from build123d import *

# Parameters (mm, degrees)
F0_R          = 11.049
F1_DEPTH      = 76.2
F1_DEPTH_BACK = 76.2
F2_W          = 61.722
F2_H          = 152.4
F3_DEPTH      = 101.6
F4_T          = -2.54


with BuildPart() as f1:
    # F0 (on Front) → F1 (new body, two sides)
    with BuildSketch(Plane.XZ) as f1_sk:
        with BuildLine():
            ThreePointArc((10.170598, -40.91247), (11.863519, -37.501733), (12.446, -33.738778))
            ThreePointArc((12.446, -33.738778), (-3.762954, -21.875259), (-10.170598, -40.91247))
            ThreePointArc((-10.170598, -40.91247), (0, -46.184778), (10.170598, -40.91247))
        make_face()
        with Locations((0, -33.738778)):
            Circle(F0_R, mode=Mode.SUBTRACT)
        with BuildLine():
            ThreePointArc((-10.170598, -40.91247), (-3.762954, -21.875259), (12.446, -33.738778))
            ThreePointArc((12.446, -33.738778), (11.863519, -37.501733), (10.170598, -40.91247))
            Line((10.170598, -40.91247), (30.861, -11.578374))
            Line((30.861, -11.578374), (0, -11.578374))
            Line((0, -11.578374), (-30.861, -11.578374))
            Line((-30.861, -11.578374), (-10.170598, -40.91247))
        make_face()
    extrude(amount=F1_DEPTH)
    extrude(f1_sk.sketch, amount=-F1_DEPTH_BACK)

    # F2 (on face) → F3 (join)
    with BuildSketch(Plane.XY.offset(-11.578374)):
        Rectangle(F2_W, F2_H)
    extrude(amount=F3_DEPTH)

    # F4
    f4_openings = [f1.faces().sort_by_distance(p)[0] for p in [
        (0, 0, 90.021626),
    ]]
    offset(amount=F4_T, openings=f4_openings)


solid = f1.part
Design review of the part built by this model. Coordinates are the model's own, in mm. A direction names the side the tool comes from. Coordinates: 2 decimals unless noted, no trailing zeros. Write each loop counter-clockwise with the first axis right and the second up, starting at its lowest first coordinate (ties: lowest second). Pieces come first, ordered by that corner, then holes. Notation, with made-up numbers: (7, -36) -> (65, -36) arc R12 ccw to (65, -24) -> close; hole circle Ø1 at (33.5, -13.75). An arc over 180 degrees is marked (long way). Write each question's results on one line, items separated by ' | '. Start each with the question number.
(1) The part is to be moulded in two halves that separate along Z. For faces 3 (the face through (-30, 23, 90.022)), 4 (the face through (0, -76.2, 36)), 5 (the face through (-1.438, 1.067, -22.784)), say which applies: pulls with the +Z half, pulls with the -Z half, needs draft (parallel to the pull), parting line crosses it, or undercut.
(2) Clearance check with flat-ended pins moving along their axes: P1, Ø12, axis at x = 18.5, y = -20.5, coming from the +Z side; P2, Ø4, axis at x = -18, y = 3.5, coming from the +Z side; P3, Ø6, axis at x = 9.5, y = 7.5, coming from the -Z side. State where each tip first meets the part, or that it passes through.
(3) Take a section at D-D on z = -5. Write out the cut boundary in (x, y).
(4) Tool access review of faces 1 (the face through (-0.167, -1.067, -46.184)), 2 (the face through (20.785, -1.031, -21.457)): name each direction out of +Z, -Z, +X, -X, +Y, -Y from which nothing blocks a thin tool from reaching the whole face with its end or side.
(5) Take a section at A-A on x = 0. Write out the cut boundary in (y, z), and give its area (3 significant figures).
(6) Take a section at C-C on y = 50. Write out the cut boundary in (x, z).
(7) For line 1 along Y through (x, z) = (-13, 8); line 2 along X through (y, z) = (-28.5, 34.5); line 3 along Z through (x, y) = (0, 1.5), list the stretches that pass through material, from the lowest coordinate up. Write a range as from..to.
(8) Take a section at B-B on z = -25.5. Write out the cut boundary in (x, y), and give its area (3 significant figures).
Results found:
1) face 3: pulls with the +Z half | face 4: needs draft | face 5: undercut
2) P1: stops at z = -16.19 | P2: stops at z = -22.57 | P3: stops at z = -44.35
3) outline: (-30.86, -76.2) -> (30.86, -76.2) -> (30.86, 76.2) -> (-30.86, 76.2) -> close; hole (-28.32, -73.66) -> (28.32, -73.66) -> (28.32, 73.66) -> (-28.32, 73.66) -> close
4) face 1: -Z, +Y, -Y | face 2: +Z
5) outline: (-76.2, -46.18) -> (76.2, -46.18) -> (76.2, -44.79) -> (-76.2, -44.79) -> close; (-76.2, -22.69) -> (76.2, -22.69) -> (76.2, 90.02) -> (73.66, 90.02) -> (73.66, -20.15) -> (-73.66, -20.15) -> (-73.66, 90.02) -> (-76.2, 90.02) -> close | area: 1,160 mm2
6) outline: (-30.86, -11.58) -> (-10.17, -40.91) arc R12.45 ccw to (10.17, -40.91) -> (30.86, -11.58) -> (30.86, 90.02) -> (28.32, 90.02) -> (28.32, -10.77) -> (13.46, -31.85) arc R13.59 ccw to (-13.46, -31.85) -> (-28.32, -10.77) -> (-28.32, 90.02) -> (-30.86, 90.02) -> close; hole circle Ø22.1 at (0, -33.74)
7) line 1: y = -76.2..-73.66, 73.66..76.2 | line 2: x = -30.86..-28.32, 28.32..30.86 | line 3: z = -46.18..-44.79, -22.69..-20.15
8) outline: (-21.04, -76.2) -> (-7.36, -76.2) -> (-7.36, 76.2) -> (-21.04, 76.2) -> close; (7.36, -76.2) -> (21.04, -76.2) -> (21.04, 76.2) -> (7.36, 76.2) -> close; hole (-17.93, -73.66) -> (-10.81, -73.66) -> (-10.81, 73.66) -> (-17.93, 73.66) -> close; hole (10.81, -73.66) -> (17.93, -73.66) -> (17.93, 73.66) -> (10.81, 73.66) -> close | area: 2,070 mm2
